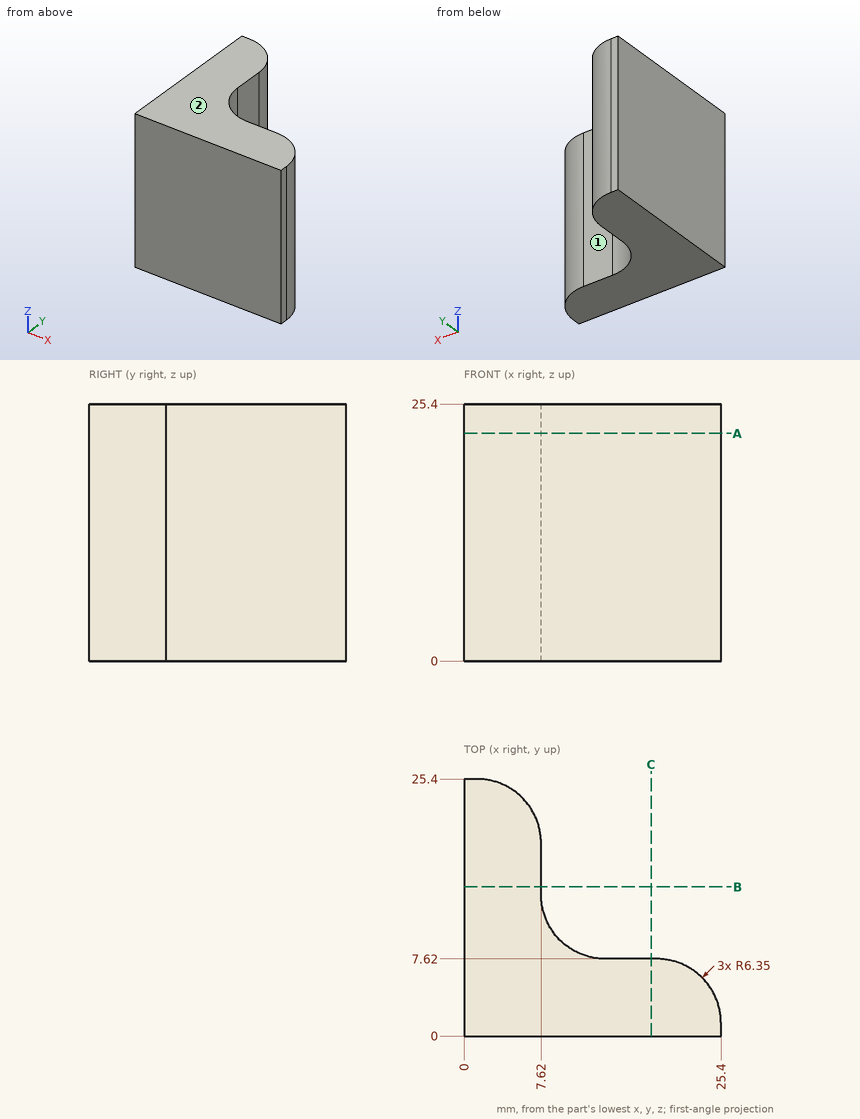
Check sheet for the drawn part. Datum: minimum x, y, z corner. Units: mm. A direction names the side the tool comes from. Coordinates: 2 decimals unless noted, no trailing zeros. Write each loop counter-clockwise with the first axis right and the second up, starting at its lowest first coordinate (ties: lowest second). Pieces come first, ordered by that corner, then holes. Notation, with made-up numbers: (61.5, 21) - (115.5, 21) arc R13 cw to (115.5, 34) - close; hole circle Ø6 at (11, -39.5). An arc over 180 degrees is marked (long way). Answer as a JSON object with one key per item and string values.
(1) Thickness scan on line 1 along X through (y, z) = (14.5, 11.25); line 2 along Y through (x, z) = (10.75, 4.75). Record the ranges inside material, lowest first.
Report:
{"line 1": "0 to 7.62", "line 2": "0 to 8.5"}
(2) Cross-section at B-B on y = 14.75. Record the cut outline in (x, z), plus the area to 3 significant figures.
Report:
{"outline": "(0, 0) - (7.62, 0) - (7.62, 25.4) - (0, 25.4) - close", "area": "194 mm^2"}
(3) Cross-section at A-A on z = 22.5. Record the cut outline in (x, y), plus the area to 3 significant figures.
Report:
{"outline": "(0, 0) - (25.4, 0) - (25.4, 1.27) arc R6.35 ccw to (19.05, 7.62) - (13.97, 7.62) arc R6.35 cw to (7.62, 13.97) - (7.62, 19.05) arc R6.35 ccw to (1.27, 25.4) - (0, 25.4) - close", "area": "320 mm^2"}
(4) Tool access check on the marked faces 1 and 2. Record the directions out of +Z, -Z, +X, -X, +Y, -Y that give a thin tool (end or side, any length) a straight path to the whole face; none if there is none.
Report:
{"face 1": "+Z, -Z, +X, +Y", "face 2": "+Z, +X, -X, +Y, -Y"}
(5) Gauge pin test, flat ends, axial feed: pin 1 Ø1 at (x, z) = (20, 12) entering from +Y; pin 2 Ø3 at (y, z) = (22.5, 16.5) entering from +X; pin 3 Ø1 at (x, z) = (5, 16.5) entering from +Y. Record the tip position at first contact, or that the pin passes through.
Report:
{"pin 1": "y = 7.6", "pin 2": "x = 7.31", "pin 3": "y = 24.52"}
